Design review of the part built by this model. Coordinates are the model's own, in mm. A direction names the side the tool comes from. Round coordinates to 2 decimals unless told otherwise and drop trailing zeros. Loops run counter-clockwise (first coordinate to the right, second up) from the corner with the lowest first, then second, coordinate; pieces in that order, holes last. Notation, with made-up numbers: (-35.75, -21.5) - (-24.75, -21.5) arc R16 ccw to (-24.75, 1.5) - close; hole circle Ø4 at (-30.75, -30). An arc over 180 degrees is marked (long way). Use one line per item in the form item = value. Start each with the question number.
(1) The part is to be moulded in two halves that separate along Y. For faces 3 (the flat face through (-55.46, 20, 10)), 4 (the conical face through (-31.341, 15.282, 3.394)), 5 (the cylindrical face through (8.33, 12.04, 3.79)), say which applies: released by +Y, released by -Y, zero draft, split by the parting line, or undercut.
(2) Machinability: for faces 1 (the flat face through (-16.438, 0, 3)), 2 (the conical face through (-21.18, 11.053, 14.415)), which of the approach directions +Z, -Z, +X, -X, +Y, -Y give a long, thin tool a straight path to every point of the face, cutting with its end or side? Answer none if there is none.
(3) Wall thickness on probe 1 along Z at (x, y) = (-25, 10.5); probe 2 along Z at (x, y) = (-12, 0); probe 3 along Y at (x, z) = (-31.5, 14.5): over which ranges is each line inside the solid? List them lowest first. Write a range as [from, to].
(4) We need section C-C, the plane x = -15. Write out the cut boundary in (y, z).
(5) For pin 1 (8 mm diameter, centred on y = -4.78, z = -5.03, fed in from -X); pin 2 (3 mm diameter, centred on x = -8, y = -12.5, fed in from +Z); pin 3 (4 mm diameter, centred on x = -32, z = 1, fed in from -Y), all flat-tipped, find the tip position at first contact; note any pin that passes through.
(6) We need section B-B, the plane x = 3.5. Write out the cut boundary in (y, z).
(7) We need section A-A, the plane y = 0. Write out the cut boundary in (x, z), then the cut area to 3 significant figures.
from build123d import *

# Parameters (mm, degrees)
F2_T        = -5
F4_D        = 5
F1_FACE_R   = 12.622695
F1_FACE_R_2 = 2.5
F5_DEPTH    = 16.4385


with BuildPart() as f1:
    # F0 (on Front) → F1 (revolve)
    with BuildSketch(Plane.XZ):
        Polygon((-55.460349, -27.133826), (0, -12.622695), (0, 0), (-55.460349, 0), align=None)
    revolve(axis=Axis((7.454347, 0, 0), (-1, 0, 0)))

    # F2
    f2_openings = [f1.faces().sort_by_distance(p)[0] for p in [
        (-55.460349, 0, 0),
    ]]
    offset(amount=F2_T, openings=f2_openings)

    # F4 (through all)
    with Locations(Plane.YZ):
        with Locations((0, 0), (-4.776739, -5.027231)):
            Hole(F4_D / 2)

    # F1_face (on face) → F5 (join, symmetric)
    with BuildSketch(Plane.YZ):
        Circle(F1_FACE_R)
        Circle(F1_FACE_R_2, mode=Mode.SUBTRACT)
        with Locations((-4.776739, -5.027231)):
            Circle(F1_FACE_R_2, mode=Mode.SUBTRACT)
    extrude(amount=F5_DEPTH, both=True)


solid = f1.part
Data:
q1.face_3 = zero draft
q1.face_4 = undercut
q1.face_5 = split by the parting line
q2.face_1 = -X
q2.face_2 = +X
q3.probe_1 = [-16.03, -9.25], [9.25, 16.03]
q3.probe_2 = [-15.76, -2.5], [2.5, 15.76]
q3.probe_3 = [-15, -6.01], [6.01, 15]
q4.outline = circle Ø33.09 at (0, 0); hole circle Ø5 at (-4.78, -5.03); hole circle Ø5 at (0, 0)
q5.pin_1 = -16.44
q5.pin_2 = 9.88
q5.pin_3 = -21.5
q6.outline = circle Ø25.25 at (0, 0); hole circle Ø5 at (-4.78, -5.03); hole circle Ø5 at (0, 0)
q7.outline = (-55.46, -27.13) - (0, -12.62) - (16.44, -12.62) - (16.44, -2.5) - (-16.44, -2.5) - (-16.44, -11.76) - (-55.46, -21.97) - close; (-55.46, 21.97) - (-16.44, 11.76) - (-16.44, 2.5) - (16.44, 2.5) - (16.44, 12.62) - (0, 12.62) - (-55.46, 27.13) - close
q7.area = 1,140 mm^2
